Input: dimensioned drawing with shaded views. Units: mm. Origin: part minimum x, y, z. A direction names the side the tool comes from. Coordinates: 2 decimals unless noted, no trailing zeros. Loops run counter-clockwise (first coordinate to the right, second up) from the corner with the lowest first, then second, coordinate; pieces in that order, holes last.
(1) Section C-C, the plane y = 44. Return loops of the section in (x, z), then the cut area to 3 significant figures.
(2) Section A-A, the plane z = 27.5. Return loops of the section in (x, y).
(3) Line query: L1, parallel to Z at x = 50.5, y = 17; L2, parallel to X at y = 16, z = 54; L3, parallel to X at y = 44, z = 7.5. Output: solid intervals per line, ascending.
(4) Set-up query: the marked faces 1 and 2. Return all of +Z, -Z, +X, -X, +Y, -Y with unobstructed straight access to the full face (end or side cutting, diameter ignored); none if empty.
(5) Section B-B, the plane x = 41. Return loops of the section in (y, z).
(6) Contact query for flat-ended pins moving along their axis: P1, Ø9, axis at x = 43, y = 38, coming from the +Z side; P2, Ø12, axis at x = 52.5, z = 52, coming from the +Y side; P3, Ø7.5, axis at y = 24.5, z = 54, coming from the +X side. Output: stop coordinate, or through.
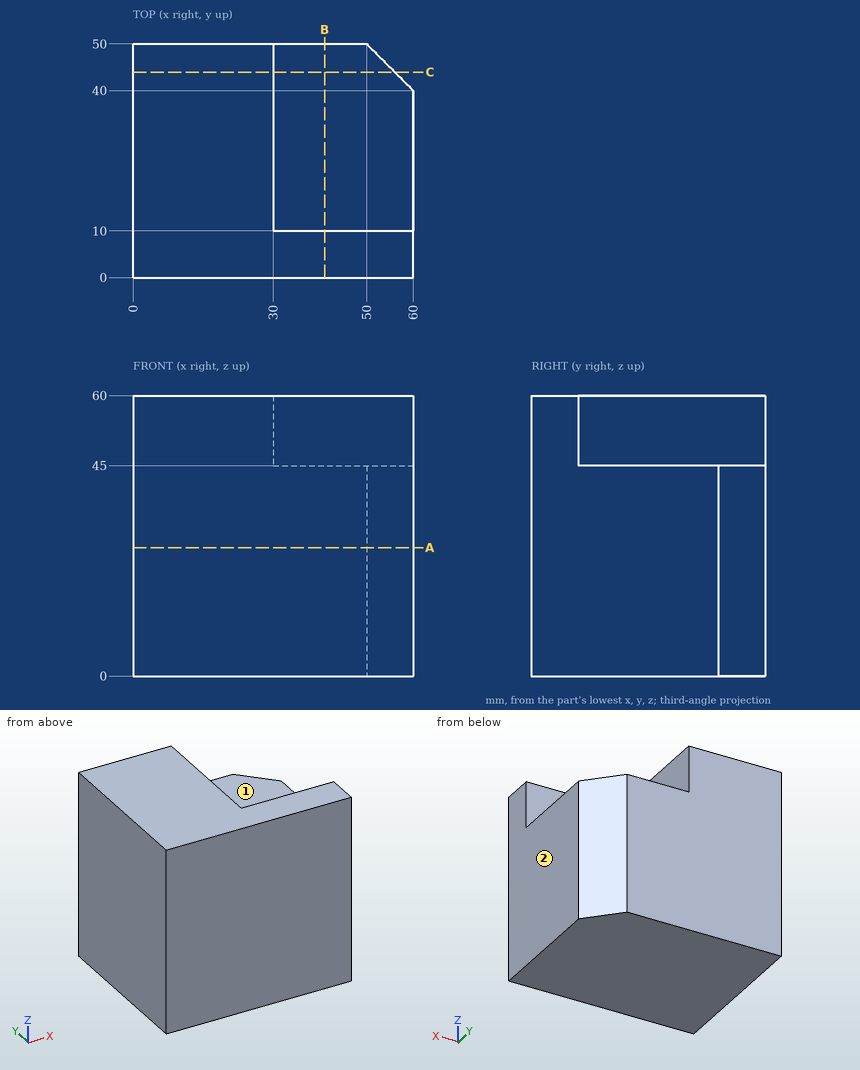
Report:
1. outline: (0, 0) - (56, 0) - (56, 45) - (30, 45) - (30, 60) - (0, 60) - close
1. area: 2,970 mm2
2. outline: (0, 0) - (60, 0) - (60, 40) - (50, 50) - (0, 50) - close
3. L1: z = 0 to 45
3. L2: x = 0 to 30
3. L3: x = 0 to 56
4. face 1: +Z, +X, +Y
4. face 2: +Z, -Z, +X, +Y, -Y
5. outline: (0, 0) - (50, 0) - (50, 45) - (10, 45) - (10, 60) - (0, 60) - close
6. P1: stops at z = 45
6. P2: stops at y = 10
6. P3: stops at x = 30
